Model file for the job. Use its own axes, mm. Face numbers are marked on the shaded views. Give positions to 0.01 mm unless a question says otherwise; leave off trailing zeros. Order: outer loops, then holes, each group sorted by start corner. A loop starts at its lowest first (then second) coordinate and runs counter-clockwise, first axis right, second up. Notation, with made-up numbers: (47.25, 71.5) - (91.25, 71.5) arc R9 cw to (91.25, 77.5) - close; hole circle Ø7 at (22.25, 51). An arc over 180 degrees is marked (long way). Use CSV: the item, a comma, the result in double quotes. Start each with the question number.
(1) Drop flat-ended pins along their axis: pin 1 Ø1.5 at (x, y) = (-16.5, 5.5) entering from +Z; pin 2 Ø1 at (y, z) = (2.5, 7) entering from +X; pin 3 Ø4 at (x, y) = (-25.5, -2.5) entering from +Z; pin 4 Ø2 at (y, z) = (3.5, 7) entering from +X. Give the stop position or say it passes through.
(2) Band-saw the part on D-D, the plane z = 7.75. Give the cut face in (x, y), then the cut area to 3 significant figures.
(3) Probe L1, parallel to Y at x = -44.45, z = 2.9; L2, parallel to Y at x = 0, z = 2.35; L3, parallel to Y at x = 0, z = 5. List the from-to ranges inside material, lowest first.
(4) Pull direction Y, two halves, no side cores. Call the marked faces 1, 2 and 3: +Y half, -Y half, draft (parallel to the pull), parting line (faces both ways), or undercut.
(5) Band-saw the part on C-C, the plane y = 0. Give the cut face in (x, z), then the cut area to 3 significant figures.
(6) Band-saw the part on B-B, the plane y = -12.7. Give the cut face in (x, z).
(7) Band-saw the part on A-A, the plane x = -44.45. Give the cut face in (y, z), then the cut area to 3 significant figures.
Autodesk Inventor part; units mm, degrees
ref_plane "YZ Plane" through (0, 0, 0) normal (1, 0, 0) x (0, 1, 0)
ref_plane "XZ Plane" through (0, 0, 0) normal (0, 1, 0) x (-1, 0, 0)
ref_plane "XY Plane" through (0, 0, 0) normal (0, 0, 1) x (1, 0, 0)
sketch "Sketch1" plane through (0, 0, 0) normal (0, 0, 1) x (1, 0, 0)
  arc A0 (-4.6555, -2.033) -> (-1.4351, 4.8731) centre (0, 0) ccw
  circle A1 centre (0, 0) radius 2.032
  arc A2 (-4.9886, -13.6592) -> (-0.3281, -7.6306) centre (0, -12.7) ccw
  circle A3 centre (0, -12.7) radius 2.032
  line L0 (-43.5629, 16.1615) -> (-4.9886, -13.6592)
  line L1 (-0.3281, -7.6306) -> (-11.9974, 1.3906)
  line L2 (-1.4351, 4.8731) -> (-39.5982, 22.6688)
  arc A4 (-39.5982, 22.6688) -> (-43.5629, 16.1615) centre (-44.45, 21.1635) ccw
  circle A5 centre (-44.45, 21.1635) radius 2.032
  line L3 (-39.5982, 22.6688) -> (-46.4155, 25.8478) construction
  line L4 (-43.5629, 16.1615) -> (-49.5141, 20.7622) construction
  line L5 (-4.6555, -2.033) -> (-11.9974, 1.3906)
  line L6 (0, 0) -> (25.4, 0) construction
  point P0 (-4.1501, -2.9296)
  point P1 (-3.0659, -4.0505)
  dimension "d0" = 10.16
  dimension "d1" = 4.064
  dimension "d7" = 10.16
  dimension "d8" = 4.064
  dimension "d9" = 12.7
  dimension "d10" = 7.62
  dimension "d11" = 3.81
  dimension "d20" = 10.16
  dimension "d21" = 4.064
  dimension "d25" = 7.62
  dimension "d29" = 44.45
  dimension "d30" = 7.62
  dimension "d31" = 3.81
  dimension "d32" = 25.4
  dimension "d33" = 25
extrude "Extrusion1" add sketch "Sketch1" along normal blind 4.826
sketch "Sketch4" plane through (0, 0, 4.826) normal (0, 0, 1) x (1, 0, 0)
  arc A0 (-4.6555, -2.033) -> (-1.4351, 4.8731) centre (0, 0) ccw
  circle A1 centre (0, 0) radius 2.032
  circle A2 centre (0, 0) radius 5.08
  point P0 (-1.4351, 4.8731)
  point P1 (-3.0659, -4.0505)
  point P2 (5.08, 0)
  point P3 (-1.4351, 4.8731)
extrude "Extrusion4" add sketch "Sketch4" along normal blind 3.81
equation "\"d8\" = d1"
equation "\"d11\" = 0.5 * d10"
properties part number "Tip Arm 2"
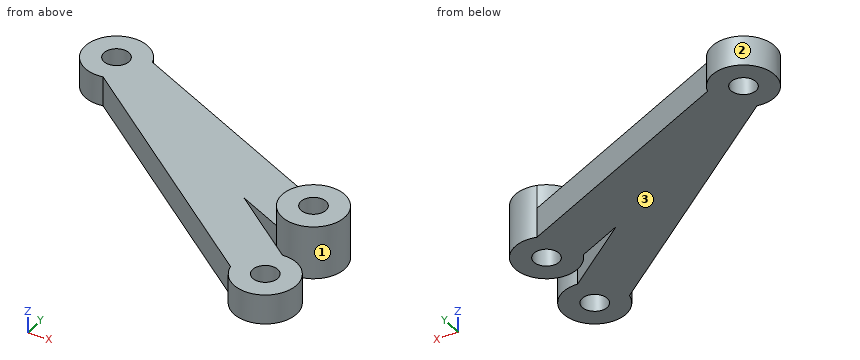
Answer block:
1,pin 1,"stops at z = 4.83"
1,pin 2,"stops at x = 4.67"
1,pin 3,"passes through"
1,pin 4,"stops at x = 4.42"
2,outline,"(-4.66, -2.03) arc R5.08 ccw (long way) to (-1.44, 4.87) arc R5.08 ccw to start; hole circle Ø4.06 at (0, 0)"
2,area,"68.1 mm2"
3,L1,"y = 16.08 to 19.13, 23.2 to 26.24"
3,L2,"y = -17.78 to -14.73, -10.67 to -7.62, -5.08 to -2.03, 2.03 to 5.08"
3,L3,"y = -5.08 to -2.03, 2.03 to 5.08"
4,face 1,"undercut"
4,face 2,"parting line"
4,face 3,"draft"
5,outline,"(-22.66, 0) - (-10.2, 0) - (-10.2, 4.83) - (-22.66, 4.83) - close; (-9.02, 0) - (-2.03, 0) - (-2.03, 8.64) - (-5.08, 8.64) - (-5.08, 4.83) - (-9.02, 4.83) - close; (2.03, 0) - (5.08, 0) - (5.08, 8.64) - (2.03, 8.64) - close"
5,area,"132 mm2"
6,outline,"(-6.23, 0) - (-2.03, 0) - (-2.03, 4.83) - (-6.23, 4.83) - close; (2.03, 0) - (5.08, 0) - (5.08, 4.83) - (2.03, 4.83) - close"
7,outline,"(16.08, 0) - (19.13, 0) - (19.13, 4.83) - (16.08, 4.83) - close; (23.2, 0) - (26.24, 0) - (26.24, 4.83) - (23.2, 4.83) - close"
7,area,"29.4 mm2"
